```python
from build123d import *

# Parameters (mm, degrees)
FILLET1_R = 0.2


with BuildPart() as part:
    # BodySke → Base-Revolve (revolve)
    with BuildSketch(Plane.XY, mode=Mode.PRIVATE) as base_revolve_sk:
        Polygon((0, 0), (0, 3.75), (0.5, 4.25), (5, 4.25), (5, 2.5), (20.555, 2.5), (21, 2.055), (21, 0), align=None)
    revolve(base_revolve_sk.sketch.rotate(Axis((-31.75, 0, 0), (1, 0, 0)), 90), axis=Axis((-31.75, 0, 0), (1, 0, 0)))

    # Fillet1
    fillet1_edges = [part.edges().sort_by_distance(p)[0] for p in [
        (5, 0, -2.5),
    ]]
    fillet(fillet1_edges, radius=FILLET1_R)


solid = part.part
```
Work out the finished part from the listing and answer in its coordinate system (mm). A direction names the side the tool comes from. Round coordinates to 2 decimals unless told otherwise and drop trailing zeros. Write each loop counter-clockwise with the first axis right and the second up, starting at its lowest first coordinate (ties: lowest second). Pieces come first, ordered by that corner, then holes.
1) Which of the six approach directions +Z, -Z, +X, -X, +Y, -Y give full straight-line access (tool end or side, diameter ignored) to faces 1 (the face through (21, 0, 0)), 2 (the face through (13, -0.1, -2.5))?
2) Consider probe 1 along X at (y, z) = (-3.5, -0.75); probe 2 along Y at (x, z) = (9.5, 0); probe 3 along Y at (x, z) = (4, -0.25). Determine where each line is inside the solid, lowest interval first.
3) A cutting plane is placed at A-A on y = 0. Determine the outline of the cut face in (x, z) (3 decimals), and give its area (3 significant figures).
4) A cutting plane is placed at D-D on x = 3. Determine the outline of the cut face in (y, z).
5) Flat-ended cylindrical pins translate along their axes: P1, Ø2, axis at x = 12, y = -2, coming from the +Z side; P2, Ø5, axis at x = 15.5, y = 1.5, coming from the -Z side; P3, Ø5, axis at y = 2.5, z = -2.5, coming from the -X side. Find the tip coordinate at first contact, or state that the pin passes through.
6) A cutting plane is placed at C-C on x = 16.5. Determine the outline of the cut face in (y, z), and give its area (3 significant figures).
Entries:
1. face 1: +Z, -Z, +X, +Y, -Y
1. face 2: +X
2. probe 1: x = 0 to 5
2. probe 2: y = -2.5 to 2.5
2. probe 3: y = -4.24 to 4.24
3. outline: (0, -3.75) - (0.5, -4.25) - (5, -4.25) - (5, -2.7) arc R0.2 cw to (5.2, -2.5) - (20.555, -2.5) - (21, -2.055) - (21, 2.055) - (20.555, 2.5) - (5.2, 2.5) arc R0.2 cw to (5, 2.7) - (5, 4.25) - (0.5, 4.25) - (0, 3.75) - close
3. area: 122 mm2
4. outline: circle Ø8.5 at (0, 0)
5. P1: stops at z = 2.29
5. P2: stops at z = -2.5
5. P3: stops at x = 0
6. outline: circle Ø5 at (0, 0)
6. area: 19.6 mm2
